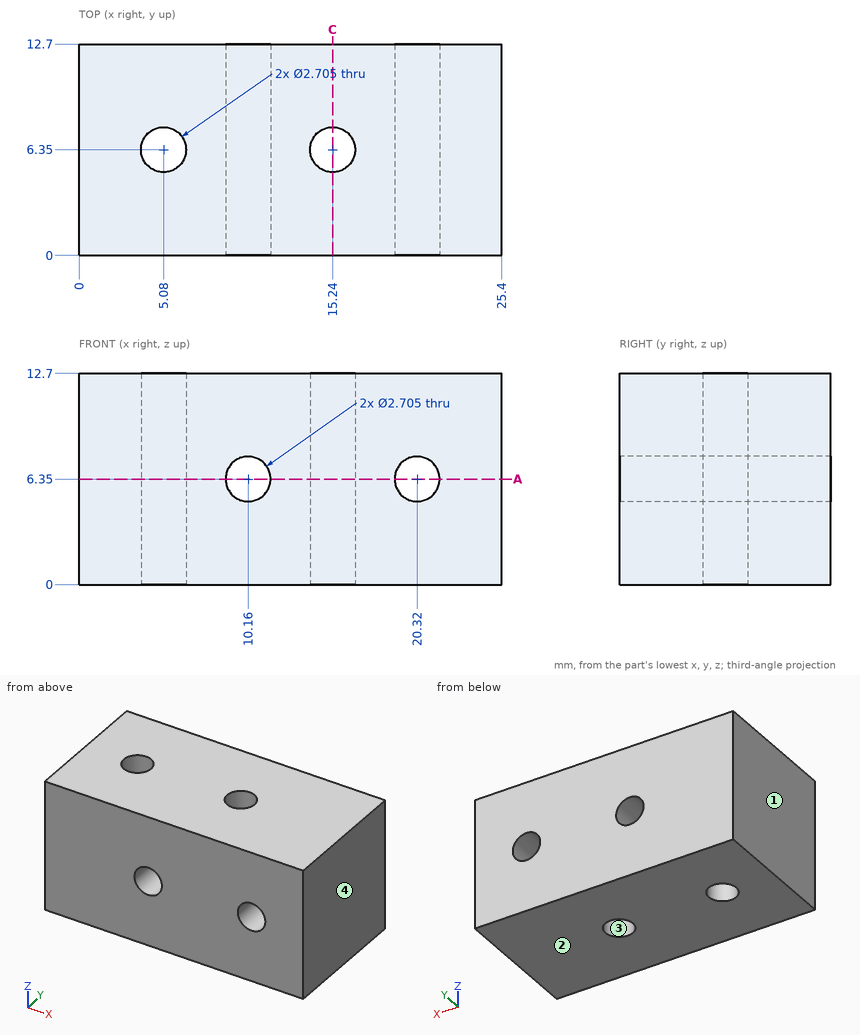
Geometry check sheet. Reference: drawing and pictorial views, mm from the part's lowest x, y, z. Round coordinates to 2 decimals unless told otherwise and drop trailing zeros. Write each loop counter-clockwise with the first axis right and the second up, starting at its lowest first coordinate (ties: lowest second). Pieces come first, ordered by that corner, then holes.
(1) Section check C-C (x = 15.24). Enter the section's corners in (y, z).
Returned:
outline: (0, 0) - (5, 0) - (5, 12.7) - (0, 12.7) - close; (7.7, 0) - (12.7, 0) - (12.7, 12.7) - (7.7, 12.7) - close
(2) Mould release check, pull along X, two halves, no side actions. Record for the marked faces 1, 2, 3 and 4: pulls with the +X half, pulls with the -X half, needs draft (parallel to the pull), parting line crosses it, or undercut.
Returned:
face 1: pulls with the -X half
face 2: needs draft
face 3: undercut
face 4: pulls with the +X half
(3) Depth check by flat-ended pin: pin 1 Ø2.5 at (x, z) = (10.16, 6.35) entering from +Y. Enter the tip coordinate at first touch or a pass-through.
Returned:
pin 1: passes through
(4) Material ranges on line 1 (X direction, y = 9, z = 6.35); line 2 (Z direction, x = 20.25, y = 0.5); line 3 (X direction, y = 6.75, z = 1), recorded low to high.
Returned:
line 1: x = 0 to 8.81, 11.51 to 18.97, 21.67 to 25.4
line 2: z = 0 to 5, 7.7 to 12.7
line 3: x = 0 to 3.79, 6.37 to 13.95, 16.53 to 25.4
(5) Section check A-A (z = 6.35). Give the number of separate pieces and of enclosed holes in the cut face, plus the area to 3 significant figures.
Returned:
separate pieces: 3
enclosed holes: 2
area: 242 mm2
